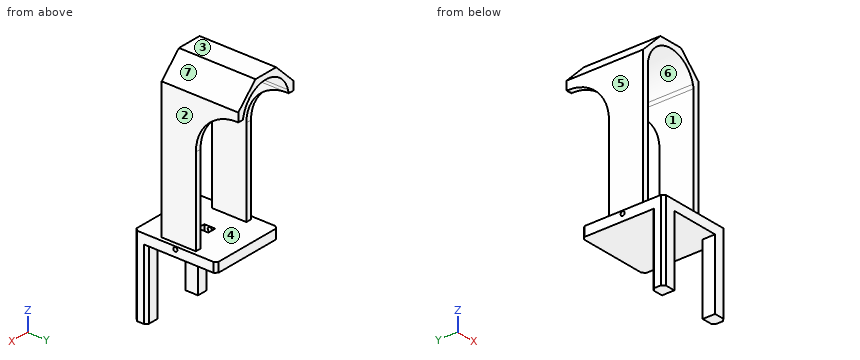
from build123d import *

# Parameters (mm, degrees)
BOSS_EXTRUDE1_DEPTH      = 5
BOSS_EXTRUDE2_DEPTH      = 56
BOSS_EXTRUDE2_2_DEPTH    = 56
BOSS_EXTRUDE3_DEPTH      = 2
BOSS_EXTRUDE3_DEPTH_BACK = 5
SKETCH9_W                = 6
SKETCH9_H                = 8
CUT_EXTRUDE3_DEPTH       = 6
CUT_EXTRUDE4_DEPTH       = 85.267431431
CUT_EXTRUDE4_DEPTH_BACK  = 85.267431431
SKETCH10_R               = 1.5
BOSS_EXTRUDE4_DEPTH      = 43.5
BOSS_EXTRUDE4_DEPTH_BACK = 12.5
SKETCH11_W               = 48
SKETCH11_H               = 115
CUT_EXTRUDE5_DEPTH       = 153.322847925
CUT_EXTRUDE6_DEPTH       = 145.966375412
CUT_EXTRUDE6_DEPTH_BACK  = 145.966375412
CHAMFER1_SIZE            = 15
CHAMFER2_SIZE            = 15


with BuildPart() as part:
    # Sketch1 → Boss-Extrude1 (new body)
    with BuildSketch(Plane.XY):
        Polygon((37.6, 51), (52, 51), (54, 53), (54, 58), (52, 60), (2, 60), (0, 58), (0, 53), (2, 51), (16.4, 51), align=None)
    extrude(amount=BOSS_EXTRUDE1_DEPTH)



with BuildPart() as body_2:
    # Sketch2 → Boss-Extrude2 (new body)
    with BuildSketch(Plane.XY.offset(-51)):
        Polygon((0, 7), (0, 2), (2, 0), (9.25, 0), (9.25, 9), (2, 9), align=None)
    extrude(amount=BOSS_EXTRUDE2_DEPTH)


with BuildPart() as body_3:
    # Sketch2 → Boss-Extrude2 2 (new body)
    with BuildSketch(Plane.XY.offset(-51)):
        Polygon((54, 2), (54, 7), (52, 9), (44.75, 9), (44.75, 0), (52, 0), align=None)
    extrude(amount=BOSS_EXTRUDE2_2_DEPTH)


with BuildPart() as part_1:
    add(part.part)

    add(body_2.part)  # Boss-Extrude3 merges body 2

    add(body_3.part)  # Boss-Extrude3 merges body 3
    # Sketch8 → Boss-Extrude3 (add, two sides: drawn at the far end of the back side and taken through both)
    with BuildSketch(Plane.XY.offset(5).offset(-BOSS_EXTRUDE3_DEPTH_BACK)):
        Polygon((0, 2), (0, 58), (2, 60), (52, 60), (54, 58), (54, 2), (52, 0), (2, 0), align=None)
    extrude(amount=BOSS_EXTRUDE3_DEPTH + BOSS_EXTRUDE3_DEPTH_BACK)

    # Sketch9 → Cut-Extrude3 (cut)
    with BuildSketch(Plane.XY.offset(7)):
        with Locations((27, 30)):
            Rectangle(SKETCH9_W, SKETCH9_H)
    extrude(amount=-CUT_EXTRUDE3_DEPTH, mode=Mode.SUBTRACT)

    # Sketch10 → Cut-Extrude4 (cut, two sides: drawn at the far end of the back side and taken through both)
    with BuildSketch(Plane.ZY.offset(-30).offset(-CUT_EXTRUDE4_DEPTH_BACK)):
        with Locations(Location((5, 30, 0), (0, 0, 270))):
            Circle(SKETCH10_R)
    extrude(amount=CUT_EXTRUDE4_DEPTH + CUT_EXTRUDE4_DEPTH_BACK, mode=Mode.SUBTRACT)

    # Sketch11 → Boss-Extrude4 (add, two sides: drawn at the far end of the back side and taken through both)
    with BuildSketch(Plane(origin=(0, 30, 0), x_dir=(1, 0, 0), z_dir=(0, 1, 0)).offset(-BOSS_EXTRUDE4_DEPTH_BACK)):
        with Locations((27, -64.5)):
            Rectangle(SKETCH11_W, SKETCH11_H)
    extrude(amount=BOSS_EXTRUDE4_DEPTH + BOSS_EXTRUDE4_DEPTH_BACK)

    # Sketch12 → Cut-Extrude5 (cut, through all)
    with BuildSketch(Plane(origin=(0, 73.5, 0), x_dir=(1, 0, 0), z_dir=(0, 1, 0))):
        with BuildLine():
            Line((7, -100.633049952), (7, -7))
            Line((7, -7), (47, -7))
            Line((47, -7), (47, -100.633049952))
            Line((47, -100.633049952), (46.318516526, -103.176380902))
            ThreePointArc((46.318516526, -103.176380902), (27, -118), (7.681483474, -103.176380902))
            Line((7.681483474, -103.176380902), (7, -100.633049952))
        make_face()
    extrude(amount=-CUT_EXTRUDE5_DEPTH, mode=Mode.SUBTRACT)

    # Sketch13 → Cut-Extrude6 (cut, two sides: drawn at the far end of the back side and taken through both)
    with BuildSketch(Plane(origin=(27, 0, 0), x_dir=(0, 0, -1), z_dir=(1, 0, 0)).offset(-CUT_EXTRUDE6_DEPTH_BACK)):
        with BuildLine():
            Line((-7, 42.5), (-70.633049952, 42.5))
            ThreePointArc((-70.633049952, 42.5), (-91.846253387, 51.286796564), (-100.633049952, 72.5))
            Line((-100.633049952, 72.5), (-100.633049952, 73.5))
            Line((-100.633049952, 73.5), (-7, 73.5))
            Line((-7, 73.5), (-7, 42.5))
        make_face()
    extrude(amount=CUT_EXTRUDE6_DEPTH + CUT_EXTRUDE6_DEPTH_BACK, mode=Mode.SUBTRACT)

    # Chamfer1
    chamfer1_edges = [part_1.edges().sort_by_distance(p)[0] for p in [
        (3, 45.5, 122),
    ]]
    chamfer(chamfer1_edges, length=CHAMFER1_SIZE)

    # Chamfer2
    chamfer2_edges = [part_1.edges().sort_by_distance(p)[0] for p in [
        (51, 45.5, 122),
    ]]
    chamfer(chamfer2_edges, length=CHAMFER2_SIZE)


solid = part_1.part
Read the model definition and answer for the solid it produces. Units are mm, in the model's axes. Face numbers are marked on the shaded views. A direction names the side the tool comes from. Round coordinates to 2 decimals unless told otherwise and drop trailing zeros. Write each loop counter-clockwise with the first axis right and the second up, starting at its lowest first coordinate (ties: lowest second). Pieces come first, ordered by that corner, then holes.
Q1. Find section C-C on y = 48.5. Determine the outline of the cut face in (x, z).
Values:
outline: (0, 0) - (54, 0) - (54, 7) - (0, 7) - close; (3, 88.63) - (7, 88.63) - (7, 100.63) - (7.68, 103.18) arc R20 cw to (46.32, 103.18) - (47, 100.63) - (47, 88.63) - (51, 88.63) - (51, 107) - (36, 122) - (18, 122) - (3, 107) - close
Q2. Find section B-B on y = 21.5. Determine the outline of the cut face in (x, z).
Values:
outline: (0, 0) - (54, 0) - (54, 7) - (51, 7) - (51, 107) - (36, 122) - (18, 122) - (3, 107) - (3, 7) - (0, 7) - close; hole (7, 7) - (47, 7) - (47, 100.63) - (46.32, 103.18) arc R20 ccw to (7.68, 103.18) - (7, 100.63) - close
Q3. Straight lines are drawn through the part: line 1 (Y direction, x = 37, z = 5); line 2 (X direction, y = 19.5, z = 22); line 3 (Z direction, x = 26, y = 46). For each, find the intervals that lie inside material, in ascending order.
Values:
line 1: y = 0 to 28.5, 31.5 to 60
line 2: x = 3 to 7, 47 to 51
line 3: z = 0 to 7, 117.97 to 122
Q4. A tool of negligible diameter and unlimited length cuts with its end or side. For the marked faces 1, 2 and 3, from which of +Z, -Z, +X, -X, +Y, -Y can it reach the whole face along a straight path? Write none if from no direction.
Values:
face 1: +Y, -Y
face 2: +Z, +X, +Y, -Y
face 3: +Z, +X, -X, +Y, -Y
Q5. Find section A-A on z = 13. Determine the outline of the cut face in (x, y), and give its area (3 significant figures).
Values:
outline: (3, 17.5) - (7, 17.5) - (7, 42.5) - (3, 42.5) - close; (47, 17.5) - (51, 17.5) - (51, 42.5) - (47, 42.5) - close
area: 200 mm2
Q6. The mould has two halves that part along Z. Classify the marked faces 4, 5, 6 and 7: released by +Z, released by -Z, zero draft, split by the parting line, or undercut.
Values:
face 4: undercut
face 5: zero draft
face 6: undercut
face 7: released by +Z
Q7. Find section D-D on z = 99. Determine the outline of the cut face in (x, y), and give its area (3 significant figures).
Values:
outline: (3, 17.5) - (7, 17.5) - (7, 62.74) - (3, 62.74) - close; (47, 17.5) - (51, 17.5) - (51, 62.74) - (47, 62.74) - close
area: 362 mm2
Q8. Flat-ended cylindrical pins translate along their axes: P1, Ø1.5, axis at y = 62.5, z = 104.5, coming from the -X side; P2, Ø5, axis at x = 10, y = 54.5, coming from the -Z side; P3, Ø7.5, axis at x = 18.5, z = 5, coming from the +Y side; P4, Ø7, axis at y = 2.5, z = -14.5, coming from the -X side. Find the tip coordinate at first contact, or state that the pin passes through.
Values:
P1: stops at x = 3
P2: stops at z = 0
P3: stops at y = 60
P4: stops at x = 0
